Design review of the part built by this model. Coordinates are the model's own, in mm. Coordinates: 2 decimals unless noted, no trailing zeros. Write each loop counter-clockwise with the first axis right and the second up, starting at its lowest first coordinate (ties: lowest second). Pieces come first, ordered by that corner, then holes.
Q1. For L1, parallel to Y at x = 116, z = 3.5; L2, parallel to X at y = 85.9, z = 25; L3, parallel to Z at x = -77, y = 86.7, list the stretches that pass through material, from the lowest coordinate up.
Q2. For pin 1 Ø1 at (x, y) = (-51.5, -56) entering from +Z, flat-tipped, find the tip position at first contact; note if it passes through.
Q3. Take a section at B-B, the plane x = -13. Write out the cut boundary in (y, z), plus the area to 3 significant figures.
Q4. Take a section at A-A, the plane y = 55.5. Write out the cut boundary in (x, z).
Q5. Take a section at C-C, the plane z = 8. State how many separate pieces and enclosed holes the cut face has, plus the area to 4 significant figures.
Autodesk Inventor part; units mm, degrees
ref_plane "YZ Plane" through (0, 0, 0) normal (1, 0, 0) x (0, 1, 0)
ref_plane "XZ Plane" through (0, 0, 0) normal (0, 1, 0) x (-1, 0, 0)
ref_plane "XY Plane" through (0, 0, 0) normal (0, 0, 1) x (1, 0, 0)
sketch "Sketch1" plane through (0, 0, 0) normal (0, 0, 1) x (1, 0, 0)
  line L0 (-130.5, -87.5) -> (130.5, -87.5)
  line L1 (130.5, -87.5) -> (130.5, 87.5)
  line L2 (130.5, 87.5) -> (-130.5, 87.5)
  line L3 (-130.5, 87.5) -> (-130.5, -87.5)
  line L4 (-130.5, -87.5) -> (130.5, 87.5) construction
  line L5 (130.5, -87.5) -> (-130.5, 87.5) construction
  point P0 (0, 0)
  dimension "d0" = 261
  dimension "d1" = 175
extrude "Extrusion1" add sketch "Sketch1" along normal blind 28
sketch "Sketch2" plane through (0, 0, 28) normal (0, 0, 1) x (1, 0, 0)
  line L0 (-127.5, 84.5) -> (-87.5, 84.5)
  line L1 (-87.5, 84.5) -> (-87.5, 44.5)
  line L2 (-87.5, 44.5) -> (-127.5, 44.5)
  line L3 (-127.5, 44.5) -> (-127.5, 84.5)
  line L4 (-127.5, 84.5) -> (-87.5, 44.5) construction
  line L5 (-87.5, 84.5) -> (-127.5, 44.5) construction
  line L6 (130.5, 87.5) -> (-130.5, 87.5)
  line L7 (-130.5, 87.5) -> (-130.5, -87.5)
  line L8 (-84.5, 84.5) -> (-44.5, 84.5)
  line L9 (-44.5, 84.5) -> (-44.5, 44.5)
  line L10 (-44.5, 44.5) -> (-84.5, 44.5)
  line L11 (-84.5, 44.5) -> (-84.5, 84.5)
  line L12 (-84.5, 84.5) -> (-44.5, 44.5) construction
  line L13 (-44.5, 84.5) -> (-84.5, 44.5) construction
  line L14 (-41.5, 84.5) -> (-1.5, 84.5)
  line L15 (-1.5, 84.5) -> (-1.5, 44.5)
  line L16 (-1.5, 44.5) -> (-41.5, 44.5)
  line L17 (-41.5, 44.5) -> (-41.5, 84.5)
  line L18 (-41.5, 84.5) -> (-1.5, 44.5) construction
  line L19 (-1.5, 84.5) -> (-41.5, 44.5) construction
  line L20 (1.5, 84.5) -> (41.5, 84.5)
  line L21 (41.5, 84.5) -> (41.5, 44.5)
  line L22 (41.5, 44.5) -> (1.5, 44.5)
  line L23 (1.5, 44.5) -> (1.5, 84.5)
  line L24 (1.5, 84.5) -> (41.5, 44.5) construction
  line L25 (41.5, 84.5) -> (1.5, 44.5) construction
  line L26 (44.5, 84.5) -> (84.5, 84.5)
  line L27 (84.5, 84.5) -> (84.5, 44.5)
  line L28 (84.5, 44.5) -> (44.5, 44.5)
  line L29 (44.5, 44.5) -> (44.5, 84.5)
  line L30 (44.5, 84.5) -> (84.5, 44.5) construction
  line L31 (84.5, 84.5) -> (44.5, 44.5) construction
  line L32 (-127.5, 41.5) -> (-87.5, 41.5)
  line L33 (-87.5, 41.5) -> (-87.5, 1.5)
  line L34 (-87.5, 1.5) -> (-127.5, 1.5)
  line L35 (-127.5, 1.5) -> (-127.5, 41.5)
  line L36 (-127.5, 41.5) -> (-87.5, 1.5) construction
  line L37 (-87.5, 41.5) -> (-127.5, 1.5) construction
  line L38 (-84.5, 41.5) -> (-44.5, 41.5)
  line L39 (-44.5, 41.5) -> (-44.5, 1.5)
  line L40 (-44.5, 1.5) -> (-84.5, 1.5)
  line L41 (-84.5, 1.5) -> (-84.5, 41.5)
  line L42 (-84.5, 41.5) -> (-44.5, 1.5) construction
  line L43 (-44.5, 41.5) -> (-84.5, 1.5) construction
  line L44 (-41.5, 41.5) -> (-1.5, 41.5)
  line L45 (-1.5, 41.5) -> (-1.5, 1.5)
  line L46 (-1.5, 1.5) -> (-41.5, 1.5)
  line L47 (-41.5, 1.5) -> (-41.5, 41.5)
  line L48 (-41.5, 41.5) -> (-1.5, 1.5) construction
  line L49 (-1.5, 41.5) -> (-41.5, 1.5) construction
  line L50 (1.5, 41.5) -> (41.5, 41.5)
  line L51 (41.5, 41.5) -> (41.5, 1.5)
  line L52 (41.5, 1.5) -> (1.5, 1.5)
  line L53 (1.5, 1.5) -> (1.5, 41.5)
  line L54 (1.5, 41.5) -> (41.5, 1.5) construction
  line L55 (41.5, 41.5) -> (1.5, 1.5) construction
  line L56 (44.5, 41.5) -> (84.5, 41.5)
  line L57 (84.5, 41.5) -> (84.5, 1.5)
  line L58 (84.5, 1.5) -> (44.5, 1.5)
  line L59 (44.5, 1.5) -> (44.5, 41.5)
  line L60 (44.5, 41.5) -> (84.5, 1.5) construction
  line L61 (84.5, 41.5) -> (44.5, 1.5) construction
  line L62 (-127.5, -1.5) -> (-87.5, -1.5)
  line L63 (-87.5, -1.5) -> (-87.5, -41.5)
  line L64 (-87.5, -41.5) -> (-127.5, -41.5)
  line L65 (-127.5, -41.5) -> (-127.5, -1.5)
  line L66 (-127.5, -1.5) -> (-87.5, -41.5) construction
  line L67 (-87.5, -1.5) -> (-127.5, -41.5) construction
  line L68 (-84.5, -1.5) -> (-44.5, -1.5)
  line L69 (-44.5, -1.5) -> (-44.5, -41.5)
  line L70 (-44.5, -41.5) -> (-84.5, -41.5)
  line L71 (-84.5, -41.5) -> (-84.5, -1.5)
  line L72 (-84.5, -1.5) -> (-44.5, -41.5) construction
  line L73 (-44.5, -1.5) -> (-84.5, -41.5) construction
  line L74 (-41.5, -1.5) -> (-1.5, -1.5)
  line L75 (-1.5, -1.5) -> (-1.5, -41.5)
  line L76 (-1.5, -41.5) -> (-41.5, -41.5)
  line L77 (-41.5, -41.5) -> (-41.5, -1.5)
  line L78 (-41.5, -1.5) -> (-1.5, -41.5) construction
  line L79 (-1.5, -1.5) -> (-41.5, -41.5) construction
  line L80 (1.5, -1.5) -> (41.5, -1.5)
  line L81 (41.5, -1.5) -> (41.5, -41.5)
  line L82 (41.5, -41.5) -> (1.5, -41.5)
  line L83 (1.5, -41.5) -> (1.5, -1.5)
  line L84 (1.5, -1.5) -> (41.5, -41.5) construction
  line L85 (41.5, -1.5) -> (1.5, -41.5) construction
  line L86 (44.5, -1.5) -> (84.5, -1.5)
  line L87 (84.5, -1.5) -> (84.5, -41.5)
  line L88 (84.5, -41.5) -> (44.5, -41.5)
  line L89 (44.5, -41.5) -> (44.5, -1.5)
  line L90 (44.5, -1.5) -> (84.5, -41.5) construction
  line L91 (84.5, -1.5) -> (44.5, -41.5) construction
  line L92 (-127.5, -44.5) -> (-87.5, -44.5)
  line L93 (-87.5, -44.5) -> (-87.5, -84.5)
  line L94 (-87.5, -84.5) -> (-127.5, -84.5)
  line L95 (-127.5, -84.5) -> (-127.5, -44.5)
  line L96 (-127.5, -44.5) -> (-87.5, -84.5) construction
  line L97 (-87.5, -44.5) -> (-127.5, -84.5) construction
  line L98 (-84.5, -44.5) -> (-44.5, -44.5)
  line L99 (-44.5, -44.5) -> (-44.5, -84.5)
  line L100 (-44.5, -84.5) -> (-84.5, -84.5)
  line L101 (-84.5, -84.5) -> (-84.5, -44.5)
  line L102 (-84.5, -44.5) -> (-44.5, -84.5) construction
  line L103 (-44.5, -44.5) -> (-84.5, -84.5) construction
  line L104 (-41.5, -44.5) -> (-1.5, -44.5)
  line L105 (-1.5, -44.5) -> (-1.5, -84.5)
  line L106 (-1.5, -84.5) -> (-41.5, -84.5)
  line L107 (-41.5, -84.5) -> (-41.5, -44.5)
  line L108 (-41.5, -44.5) -> (-1.5, -84.5) construction
  line L109 (-1.5, -44.5) -> (-41.5, -84.5) construction
  line L110 (1.5, -44.5) -> (41.5, -44.5)
  line L111 (41.5, -44.5) -> (41.5, -84.5)
  line L112 (41.5, -84.5) -> (1.5, -84.5)
  line L113 (1.5, -84.5) -> (1.5, -44.5)
  line L114 (1.5, -44.5) -> (41.5, -84.5) construction
  line L115 (41.5, -44.5) -> (1.5, -84.5) construction
  line L116 (44.5, -44.5) -> (84.5, -44.5)
  line L117 (84.5, -44.5) -> (84.5, -84.5)
  line L118 (84.5, -84.5) -> (44.5, -84.5)
  line L119 (44.5, -84.5) -> (44.5, -44.5)
  line L120 (44.5, -44.5) -> (84.5, -84.5) construction
  line L121 (84.5, -44.5) -> (44.5, -84.5) construction
  line L122 (87.5, 84.5) -> (127.5, 84.5)
  line L123 (127.5, 84.5) -> (127.5, 44.5)
  line L124 (127.5, 44.5) -> (87.5, 44.5)
  line L125 (87.5, 44.5) -> (87.5, 84.5)
  line L126 (87.5, 84.5) -> (127.5, 44.5) construction
  line L127 (127.5, 84.5) -> (87.5, 44.5) construction
  line L128 (87.5, 41.5) -> (127.5, 41.5)
  line L129 (127.5, 41.5) -> (127.5, 1.5)
  line L130 (127.5, 1.5) -> (87.5, 1.5)
  line L131 (87.5, 1.5) -> (87.5, 41.5)
  line L132 (87.5, 41.5) -> (127.5, 1.5) construction
  line L133 (127.5, 41.5) -> (87.5, 1.5) construction
  line L134 (87.5, -1.5) -> (127.5, -1.5)
  line L135 (127.5, -1.5) -> (127.5, -41.5)
  line L136 (127.5, -41.5) -> (87.5, -41.5)
  line L137 (87.5, -41.5) -> (87.5, -1.5)
  line L138 (87.5, -1.5) -> (127.5, -41.5) construction
  line L139 (127.5, -1.5) -> (87.5, -41.5) construction
  line L140 (87.5, -44.5) -> (127.5, -44.5)
  line L141 (127.5, -44.5) -> (127.5, -84.5)
  line L142 (127.5, -84.5) -> (87.5, -84.5)
  line L143 (87.5, -84.5) -> (87.5, -44.5)
  line L144 (87.5, -44.5) -> (127.5, -84.5) construction
  line L145 (127.5, -44.5) -> (87.5, -84.5) construction
  point P0 (0, 0)
  point P1 (-107.5, 64.5)
  point P2 (-64.5, 64.5)
  point P3 (-21.5, 64.5)
  point P4 (21.5, 64.5)
  point P5 (64.5, 64.5)
  point P6 (-107.5, 21.5)
  point P7 (-64.5, 21.5)
  point P8 (-21.5, 21.5)
  point P9 (21.5, 21.5)
  point P10 (64.5, 21.5)
  point P11 (-107.5, -21.5)
  point P12 (-64.5, -21.5)
  point P13 (-21.5, -21.5)
  point P14 (21.5, -21.5)
  point P15 (64.5, -21.5)
  point P16 (-107.5, -64.5)
  point P17 (-64.5, -64.5)
  point P18 (-21.5, -64.5)
  point P19 (21.5, -64.5)
  point P20 (64.5, -64.5)
  point P21 (107.5, 64.5)
  point P22 (107.5, 21.5)
  point P23 (107.5, -21.5)
  point P24 (107.5, -64.5)
  dimension "d4" = 40
  dimension "d5" = 3
  dimension "d6" = 3
  dimension "d7" = 40
  dimension "d10" = 43
  dimension "d13" = 43
extrude "Extrusion2" cut sketch "Sketch2" against normal blind 25
sketch "Sketch3" plane through (-130.5, 87.5, 0) normal (0, 1, 0) x (1, 0, 0)
  line L0 (46, -28) -> (46, -3) construction
  line L1 (43, -28) -> (43, -3) construction
  line L2 (43, -28) -> (43, -3)
  line L3 (43, -25) -> (46, -25) construction
  line L4 (46, -28) -> (46, -3)
  line L5 (261, -28) -> (0, -28)
  circle A0 centre (53.5, -25) radius 1.65
  circle A1 centre (35.5, -25) radius 1.65
  line L6 (172, -28) -> (172, -3) construction
  line L7 (175, -28) -> (175, -3) construction
  circle A2 centre (225.5, -25) radius 1.65
  circle A3 centre (207.5, -25) radius 1.65
  line L8 (261, 0) -> (261, -28)
  point P0 (130.5, 0)
  point P1 (44.5, -25)
  dimension "d20" = 3
  dimension "d21" = 3.3
  dimension "d22" = 9
  dimension "d23" = 3.3
  dimension "d24" = 9
  dimension "d25" = 3.3
  dimension "d31" = 3.3
  dimension "d35" = 18
  dimension "d36" = 35.5
extrude "Extrusion3" cut sketch "Sketch3" against normal blind 10
equation "\"d0\" = box_length"
equation "\"d1\" = box_width"
equation "\"d2\" = hole_height + wall"
equation "\"d4\" = hole"
equation "\"d5\" = wall"
equation "\"d6\" = wall"
equation "\"d7\" = hole"
equation "\"d10\" = hole + wall"
equation "\"d13\" = hole + wall"
equation "\"d16\" = hole_height"
equation "\"d23\" = d21"
equation "\"d25\" = d21"
equation "\"d31\" = d25"
equation "\"hole\" = 40"
equation "\"wall\" = 3"
equation "\"hole_height\" = 25"
properties part number "RatPelletBox_v03"
Responses:
1. L1: y = -87.5 to -84.5, -44.5 to -41.5, -1.5 to 1.5, 41.5 to 44.5, 84.5 to 87.5
1. L2: x = -130.5 to -96.65, -93.35 to -78.65, -75.35 to 75.35, 78.65 to 93.35, 96.65 to 130.5
1. L3: z = 0 to 23.35, 26.65 to 28
2. pin 1: stops at z = 3
3. outline: (-87.5, 0) - (87.5, 0) - (87.5, 28) - (84.5, 28) - (84.5, 3) - (44.5, 3) - (44.5, 28) - (41.5, 28) - (41.5, 3) - (1.5, 3) - (1.5, 28) - (-1.5, 28) - (-1.5, 3) - (-41.5, 3) - (-41.5, 28) - (-44.5, 28) - (-44.5, 3) - (-84.5, 3) - (-84.5, 28) - (-87.5, 28) - close
3. area: 900 mm2
4. outline: (-130.5, 0) - (130.5, 0) - (130.5, 28) - (127.5, 28) - (127.5, 3) - (87.5, 3) - (87.5, 28) - (84.5, 28) - (84.5, 3) - (44.5, 3) - (44.5, 28) - (41.5, 28) - (41.5, 3) - (1.5, 3) - (1.5, 28) - (-1.5, 28) - (-1.5, 3) - (-41.5, 3) - (-41.5, 28) - (-44.5, 28) - (-44.5, 3) - (-84.5, 3) - (-84.5, 28) - (-87.5, 28) - (-87.5, 3) - (-127.5, 3) - (-127.5, 28) - (-130.5, 28) - close
5. separate pieces: 1
5. enclosed holes: 24
5. area: 7,275 mm2
